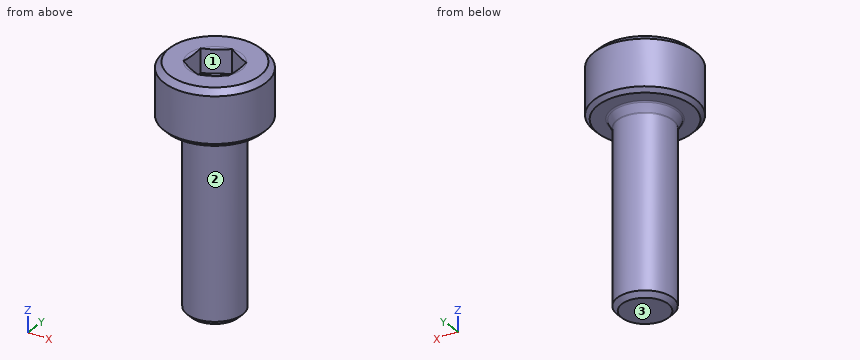
```python
from build123d import *

# Parameters (mm, degrees)
CUT_EXTRUDE1_DEPTH = 1.3


with BuildPart() as part:
    # Sketch1 → Revolve1 (revolve)
    with BuildSketch(Plane(origin=(0, 0, 0), x_dir=(0, 0, -1), z_dir=(1, 0, 0))):
        with BuildLine():
            Line((0, 0), (0, 2.45))
            Line((0, 2.45), (0.3, 2.75))
            Line((0.3, 2.75), (2.785, 2.75))
            Line((2.785, 2.75), (3, 2.535))
            Line((3, 2.535), (3, 1.8))
            ThreePointArc((3, 1.8), (3.015193643, 1.74701055), (3.056157637, 1.710123155))
            Line((3.056157637, 1.710123155), (3.466157637, 1.510123155))
            ThreePointArc((3.466157637, 1.510123155), (3.48750205, 1.50256365), (3.51, 1.5))
            Line((3.51, 1.5), (12.75, 1.5))
            Line((12.75, 1.5), (13, 1.25))
            Line((13, 1.25), (13, 0))
            Line((13, 0), (0, 0))
        make_face()
    revolve(axis=Axis((0, 0, 0), (0, 0, -1)))

    # Sketch2 → Cut-Extrude1 (cut)
    with BuildSketch(Plane.XY):
        Polygon((0, 1.443375673), (-1.25, 0.721687836), (-1.25, -0.721687836), (0, -1.443375673), (1.25, -0.721687836), (1.25, 0.721687836), align=None)
    extrude(amount=-CUT_EXTRUDE1_DEPTH, mode=Mode.SUBTRACT)

    # Sketch3 → Cut-Revolve2 (revolve, cut)
    with BuildSketch(Plane(origin=(0, 0, 0), x_dir=(0, 0, -1), z_dir=(1, 0, 0))):
        Polygon((1.3, 0), (1.3, 1.25), (2.021687836, 0), align=None)
    revolve(axis=Axis((0, 0, -1.3), (0, 0, -1)), mode=Mode.SUBTRACT)

    # Sketch4 → Cut-Revolve3 (revolve, cut)
    with BuildSketch(Plane(origin=(0, 0, 0), x_dir=(0, 0, -1), z_dir=(1, 0, 0))):
        Polygon((0, 1.443375673), (0, 1.25), (0.051814855, 1.25), align=None)
    revolve(axis=Axis((0, 0, 0), (0, 0, -1)), mode=Mode.SUBTRACT)


solid = part.part
```
The model under review builds one solid part; all positions refer to its coordinate system, in mm. Face numbers are marked on the shaded views. Round coordinates to 2 decimals unless told otherwise and drop trailing zeros. Order: outer loops, then holes, each group sorted by start corner. A loop starts at its lowest first (then second) coordinate and runs counter-clockwise, first axis right, second up.
Item 1: Draft analysis for pull direction Y (two halves, no side actions). For the marked faces 1, 2 and 3, state which applies: released by +Y, released by -Y, zero draft, split by the parting line, or undercut.
Working result:
face 1: undercut
face 2: split by the parting line
face 3: zero draft
Item 2: Add section A-A, the plane z = -8.25. State the section outline as (x, y) points, and give its area (3 significant figures).
Working result:
outline: circle Ø3 at (0, 0)
area: 7.07 mm2
Item 3: For pin 1 (3 mm diameter, centred on x = 2, z = -9.5, fed in from +Y), flat-tipped, find the tip position at first contact; note if it passes through.
Working result:
pin 1: stops at y = 1.41
Item 4: Add section B-B, the plane z = -1.75. State the section outline as (x, y) points, and give its area (3 significant figures).
Working result:
outline: circle Ø5.5 at (0, 0); hole circle Ø0.94 at (0, 0)
area: 23.1 mm2
Item 5: To check wall thickness, follow probe 1 along Z at (x, y) = (1.85, 1); probe 2 along Z at (x, y) = (0.95, -0.8); probe 3 along Y at (x, z) = (-0.95, -7.25). State the ranges of each line that lie inside material, in increasing order.
Working result:
probe 1: z = -3 to 0
probe 2: z = -13 to -1.3
probe 3: y = -1.16 to 1.16
